Check sheet for the modelled part. Datum: model origin and axes. Units: mm. A direction names the side the tool comes from. Round coordinates to 2 decimals unless told otherwise and drop trailing zeros. Write each loop counter-clockwise with the first axis right and the second up, starting at its lowest first coordinate (ties: lowest second). Pieces come first, ordered by that corner, then holes. Notation, with made-up numbers: M 11.5,46.5 L 20.5,46.5 A19 ccw 20.5,79.5 Z; hole C -31.75,71 d10. An arc over 180 degrees is marked long. Put each result on its own line as item: value.
```python
from build123d import *

# Parameters (mm, degrees)
CORTE_EXTRUS_O1_START            = -6.25
CORTE_EXTRUS_O1_OUTLINE_R        = 4.55
CORTE_EXTRUS_O1_DEPTH            = 6.25
CORTE_EXTRUS_O1_START_2          = -15
CORTE_EXTRUS_O1_2_OUTLINE_R      = 4.45
CORTE_EXTRUS_O1_2_DEPTH          = 12.640520374
CORTE_EXTRUS_O1_3_DEPTH          = 4.2
CORTE_EXTRUS_O1_4_DEPTH          = 3.890520374
CORTE_EXTRUS_O1_START_3          = 2.5
CORTE_EXTRUS_O1_5_DEPTH          = 3.5
CORTE_EXTRUS_O2_REACH            = 23.61
CORTE_EXTRUS_O3_REACH            = 19.848
FURO_DE_DI_METRO_2_5_2_5_1_D     = 2.5
FURO_DE_DI_METRO_2_5_2_5_1_DEPTH = 15
FURO_DE_DI_METRO_2_5_2_5_2_D     = 2.5
CHANFRO1_SIZE                    = 0.25
FILETE1_R                        = 0.25


with BuildPart() as part:
    # Corte-extrusão1: read off the stored shape, not the designer's step
    # Corte-extrusão1 outline → Corte-extrusão1 (new body)
    with BuildSketch(Plane.XZ.offset(15).offset(CORTE_EXTRUS_O1_START)):
        with BuildLine():
            Line((10.75, -2.331844763), (10.75, 2.331844763))
            ThreePointArc((10.75, 2.331844763), (-11, 0), (10.75, -2.331844763))
        make_face()
        Circle(CORTE_EXTRUS_O1_OUTLINE_R, mode=Mode.SUBTRACT)
    extrude(amount=CORTE_EXTRUS_O1_DEPTH)



with BuildPart() as body_2:
    # Corte-extrus_o1 2 outline → Corte-extrus_o1 2 (new body)
    with BuildSketch(Plane.XZ.offset(15).offset(CORTE_EXTRUS_O1_START_2)):
        Circle(CORTE_EXTRUS_O1_2_OUTLINE_R)
        Polygon((2.5, -1.443375673), (0, -2.886751346), (-2.5, -1.443375673), (-2.5, 1.443375673), (0, 2.886751346), (2.5, 1.443375673), align=None, mode=Mode.SUBTRACT)
    extrude(amount=CORTE_EXTRUS_O1_2_DEPTH)


with BuildPart() as part_1:
    add(part.part)

    add(body_2.part)  # Corte-extrus_o1 3 merges body 2
    # Corte-extrus_o1 3 outline → Corte-extrus_o1 3 (add)
    with BuildSketch(Plane.XZ.offset(15).offset(CORTE_EXTRUS_O1_START)):
        with BuildLine():
            Line((2.5, -0.381), (2.5, -1.443375673))
            Line((2.5, -1.443375673), (0, -2.886751346))
            Line((0, -2.886751346), (-2.5, -1.443375673))
            Line((-2.5, -1.443375673), (-2.5, 1.443375673))
            Line((-2.5, 1.443375673), (0, 2.886751346))
            Line((0, 2.886751346), (2.5, 1.443375673))
            Line((2.5, 1.443375673), (2.5, 0.381))
            Line((2.5, 0.381), (4.534020181, 0.381))
            ThreePointArc((4.534020181, 0.381), (-4.55, 0), (4.534020181, -0.381))
            Line((4.534020181, -0.381), (2.5, -0.381))
        make_face()
    extrude(amount=CORTE_EXTRUS_O1_3_DEPTH)

    # Corte-extrus_o1 4 outline → Corte-extrus_o1 4 (add)
    with BuildSketch(Plane.XZ.offset(15).offset(CORTE_EXTRUS_O1_START)):
        with BuildLine():
            ThreePointArc((4.433659775, 0.381), (4.45, 0), (4.433659775, -0.381))
            Line((4.433659775, -0.381), (4.534020181, -0.381))
            ThreePointArc((4.534020181, -0.381), (4.55, 0), (4.534020181, 0.381))
            Line((4.534020181, 0.381), (4.433659775, 0.381))
        make_face()
    extrude(amount=CORTE_EXTRUS_O1_4_DEPTH)

    # Corte-extrus_o1 5 outline → Corte-extrus_o1 5 (add)
    with BuildSketch(Plane.YZ.offset(CORTE_EXTRUS_O1_START_3)):
        with BuildLine():
            Line((-12.640520474, -0.381), (-12.640520474, 0.381))
            ThreePointArc((-12.640520474, 0.381), (-12.7, 0), (-12.640520474, -0.381))
        make_face()
    extrude(amount=CORTE_EXTRUS_O1_5_DEPTH)

    # Corte-extrusão2: up to this cone (the profile starts outside it)
    corte_extrus_o2_end = Plane(origin=(10.673877, -11.45, 0), z_dir=(1, 0, 0)).offset(-1.423876) * Cone(1e-06, 26.957754, 26.957753, align=(Align.CENTER, Align.CENTER, Align.MIN), mode=Mode.PRIVATE)
    # Esboço2 → Corte-extrusão2 (cut, up to the surface)
    with BuildSketch(Plane.XZ.offset(15), mode=Mode.PRIVATE) as corte_extrus_o2_sk1:
        with BuildLine():
            Line((10.75, -0.25), (10.75, 0.25))
            Line((10.75, 0.25), (10.588388348, 0.088388348))
            ThreePointArc((10.588388348, 0.088388348), (10.551776695, 0), (10.588388348, -0.088388348))
            Line((10.588388348, -0.088388348), (10.75, -0.25))
        make_face()
    corte_extrus_o2_tool1 = extrude(corte_extrus_o2_sk1.sketch, amount=-CORTE_EXTRUS_O2_REACH, mode=Mode.PRIVATE) - corte_extrus_o2_end
    add(corte_extrus_o2_tool1.solids().sort_by_distance((10.673877, -15, 0))[0], mode=Mode.SUBTRACT)

    # Corte-extrusão3: up to this cone (the profile starts outside it)
    corte_extrus_o3_end = Plane(origin=(10.673877, -11.45, 0), z_dir=(1, 0, 0)).offset(-1.423876) * Cone(1e-06, 23.195754, 23.195753, align=(Align.CENTER, Align.CENTER, Align.MIN), mode=Mode.PRIVATE)
    # Esboço3 → Corte-extrusão3 (cut, up to the surface)
    with BuildSketch(Plane(origin=(0, -8.75, 0), x_dir=(-1, 0, 0), z_dir=(0, 1, 0)), mode=Mode.PRIVATE) as corte_extrus_o3_sk1:
        with BuildLine():
            Line((-10.75, 0.25), (-10.75, -0.25))
            Line((-10.75, -0.25), (-10.588388348, -0.088388348))
            ThreePointArc((-10.588388348, -0.088388348), (-10.551776695, 0), (-10.588388348, 0.088388348))
            Line((-10.588388348, 0.088388348), (-10.75, 0.25))
        make_face()
    corte_extrus_o3_tool1 = extrude(corte_extrus_o3_sk1.sketch, amount=-CORTE_EXTRUS_O3_REACH, mode=Mode.PRIVATE) - corte_extrus_o3_end
    add(corte_extrus_o3_tool1.solids().sort_by_distance((10.673877, -8.75, 0))[0], mode=Mode.SUBTRACT)

    # Esboço4 → Corte-Revolução1 (revolve, cut)
    with BuildSketch(Plane(origin=(0, 0, 0), x_dir=(-1, 0, 0), z_dir=(0, 0, -1)), mode=Mode.PRIVATE) as corte_revolu_o1_sk:
        Polygon((-10.75, -9.95), (-10.75, -11.45), (-2.5, -11.45), (-2.5, -10.2), (-10.5, -10.2), align=None)
    revolve(corte_revolu_o1_sk.sketch.rotate(Axis((10.75, -11.45, 0), (-1, 0, 0)), 9.594068227), axis=Axis((10.75, -11.45, 0), (-1, 0, 0)), mode=Mode.SUBTRACT)

    # Furo de diâmetro Ø2.5 (2.5)1
    with Locations(Plane(origin=(0, -15, 0), x_dir=(-1, 0, 0), z_dir=(0, -1, 0))):
        with Locations((-4, -6.92820323), (8, 0)):
            Hole(FURO_DE_DI_METRO_2_5_2_5_1_D / 2, depth=FURO_DE_DI_METRO_2_5_2_5_1_DEPTH)

    # Furo de diâmetro Ø2.5 (2.5)2 (through all)
    with Locations(Plane(origin=(0, -8.75, 0), x_dir=(1, 0, 0), z_dir=(0, 1, 0))):
        with Locations((-4, -6.92820323), (4, 6.92820323), (-4, 6.92820323)):
            Hole(FURO_DE_DI_METRO_2_5_2_5_2_D / 2)

    # Chanfro1
    chanfro1_edges = [part_1.edges().sort_by_distance(p)[0] for p in [
        (1.25, 0, 2.165063509),
        (-1.25, 0, 2.165063509),
        (-2.5, 0, 0),
        (-1.25, 0, -2.165063509),
        (1.25, 0, -2.165063509),
        (2.5, 0, 0),
        (-4.55, -15, 0),
        (-9.25, -8.75, 0),
        (-9.25, -15, 0),
        (2.75, -8.75, 6.92820323),
        (2.75, -15, 6.92820323),
        (-2.75, -8.75, -6.92820323),
        (-2.75, -15, -6.92820323),
        (5.25, -8.75, -6.92820323),
        (5.25, -15, -6.92820323),
        (-2.75, -8.75, 6.92820323),
        (-2.75, -15, 6.92820323),
    ]]
    chamfer(chanfro1_edges, length=CHANFRO1_SIZE)

    # Filete1
    # the kernel refuses this fillet: 0.25 mm, written as the material it takes off along each edge
    with BuildSketch(Plane(origin=(10.75, -8.75, -3.394344763), x_dir=(-1, 0, 0), z_dir=(0, 0, 1)), Plane(origin=(10.75, -15, -0.375), x_dir=(0, 1, 0), z_dir=(0, 0, 1)), Plane(origin=(10.75, -15, -3.394344763), x_dir=(0, 1, 0), z_dir=(0, 0, 1)), Plane(origin=(10.75, -8.75, -0.375), x_dir=(-1, 0, 0), z_dir=(0, 0, 1))) as filete1_piece_1:
        with BuildLine():
            CenterArc((FILETE1_R, FILETE1_R), FILETE1_R, 180, 90)
            Line((0, FILETE1_R), (0, 0))
            Line((0, 0), (FILETE1_R, 0))
        make_face()
    extrude(amount=3.769344763, mode=Mode.SUBTRACT)
    with BuildSketch(Plane(origin=(0, -8.75, 0), x_dir=(0.9877835196921515, 0, 0.15583234011136815), z_dir=(0.15583234011136815, 0, -0.9877835196921515))) as filete1_piece_2:
        with BuildLine():
            CenterArc((11 - FILETE1_R, FILETE1_R), FILETE1_R, 270, 90)
            Line((11, FILETE1_R), (11, 0))
            Line((11, 0), (11 - FILETE1_R, 0))
        make_face()
    revolve(axis=Axis((0, -8.75, 0), (0, -1, 0)), revolution_arc=342.069855141, mode=Mode.SUBTRACT)
    with BuildSketch(Plane(origin=(0, -15, 0), x_dir=(0.9877835196921515, 0, 0.15583234011136815), z_dir=(0.15583234011136815, 0, -0.9877835196921515))) as filete1_piece_3:
        with BuildLine():
            CenterArc((11 - FILETE1_R, -FILETE1_R), FILETE1_R, 0, 90)
            Line((11 - FILETE1_R, 0), (11, 0))
            Line((11, 0), (11, -FILETE1_R))
        make_face()
    revolve(axis=Axis((0, -15, 0), (0, -1, 0)), revolution_arc=342.069855141, mode=Mode.SUBTRACT)


solid = part_1.part
```
1. Cross-section at B-B (y = -11.45). Enter the section's corners in (x, z).
Computed values:
outline: M -2.5,-1.44 L -2.5,1.44 L 0,2.89 L 2.5,1.44 L 2.5,1.25 L 10.5,1.25 L 10.75,1.5 L 10.75,2.33 A11 ccw long 10.75,-2.33 L 10.75,-1.5 L 10.5,-1.25 L 2.5,-1.25 L 2.5,-1.44 L 0,-2.89 Z; hole C -8,0 d2.5; hole C -4,-6.93 d2.5; hole C -4,6.93 d2.5; hole C 4,-6.93 d2.5; hole C 4,6.93 d2.5
2. Release check for a two-part mould opening along Y. For faces 1 (the cylindrical face through (6.56, -10.23, 0.28)), 2 (the cylindrical face through (4.245, -4.314, 1.337)), 3 (the flat face through (4.45, -15, -2.24)) record: +Y half, -Y half, draft (parallel to the pull), parting line (faces both ways), or undercut.
Computed values:
face 1: undercut
face 2: draft
face 3: -Y half
3. Depth check by flat-ended pin: pin 1 Ø2 at (x, y) = (-8.5, -11.5) entering from -Z; pin 2 Ø5 at (x, y) = (-2.5, -5) entering from +Z; pin 3 Ø2 at (x, z) = (4, 6.93) entering from -Y; pin 4 Ø1 at (x, z) = (2.5, -7) entering from +Y. Enter the tip coordinate at first touch or a pass-through.
Computed values:
pin 1: stops at z = -8.05
pin 2: stops at z = 4.45
pin 3: passes through
pin 4: stops at y = -8.75
4. Scan lines: probe 1 along X at (y, z) = (-9.5, 7.5); probe 2 along Z at (x, y) = (5, -11.45); probe 3 along X at (y, z) = (-13.75, -1). Record each from-to range of solid material in increasing order.
Computed values:
probe 1: x = -8.05 to -5.11, -2.89 to 2.89, 5.11 to 8.05
probe 2: z = -9.8 to -7.68, -6.18 to -1.25, 1.25 to 6.18, 7.68 to 9.8
probe 3: x = -10.95 to -8.75, -7.25 to -4.44, 4.44 to 10.75
5. Cross-section at A-A (y = -7.25). Enter the section's corners in (x, z), then the cut area to 3 significant figures.
Computed values:
outline: C 0,0 d8.9; hole M -2.5,-1.44 L 0,-2.89 L 2.5,-1.44 L 2.5,1.44 L 0,2.89 L -2.5,1.44 Z
area: 40.6 mm2
6. Cross-section at C-C (z = 6.25). Count the separate pieces of the cut face and the enclosed holes in it, then the cut area to 3 significant figures.
Computed values:
separate pieces: 3
enclosed holes: 0
area: 86.5 mm2
7. Access from +Z, -Z, +X, -X, +Y, -Y to the whole of each face (thin tool, end or side, straight path). Record for faces 4 (the flat face through (-1.29, -0.12, -2.29)), 5 (the flat face through (2.5, -5, 0)), 6 (the flat face through (10.75, -12, -2)).
Computed values:
face 4: +Y
face 5: +Y, -Y
face 6: +Z, -Z, +X, +Y, -Y
